from build123d import *

# Parameters (mm, degrees)
SKETCH_1_R          = 1.75
EXTRUDE_1_DEPTH     = 6
FILLET_1_R          = 3
SKETCH_2_R          = 0.5
CUT_EXTRUDE_1_DEPTH = 7


with BuildPart() as part:
    # Эскиз1 → Бобышка-Вытянуть1 (new body)
    with BuildSketch(Plane(origin=(0, 0, 0), x_dir=(1, 0, 0), z_dir=(0, 1, 0))):
        with BuildLine():
            Line((-3.991673782, 0), (4.008326218, 0))
            ThreePointArc((4.008326218, 0), (5.472792312, 3.535533906), (9.008326218, 5))
            Line((9.008326218, 5), (22.681786604, 5))
            ThreePointArc((22.681786604, 5), (25.510213728, 3.828427125), (26.681786604, 1))
            Line((26.681786604, 1), (29.008326218, 1))
            Line((29.008326218, 1), (53.280650212, 9.83440345))
            ThreePointArc((53.280650212, 9.83440345), (56.269012599, 16.242967271), (49.860448779, 19.231329658))
            Line((49.860448779, 19.231329658), (27.245056411, 11))
            Line((27.245056411, 11), (4.445056411, 11))
            ThreePointArc((4.445056411, 11), (-1.63962848, 6.931421506), (-3.991673782, 0))
        make_face()
        with Locations((51.570549496, 14.532866554)):
            Circle(SKETCH_1_R, mode=Mode.SUBTRACT)
        with Locations((29.781786604, 6)):
            Circle(SKETCH_1_R, mode=Mode.SUBTRACT)
    extrude(amount=EXTRUDE_1_DEPTH)

    # Скругление1
    fillet_1_edges = [part.edges().sort_by_distance(p)[0] for p in [
        (29.008326218, 3, -1),
    ]]
    fillet(fillet_1_edges, radius=FILLET_1_R)

    # Эскиз2 → Вырез-Вытянуть1 (cut, through all)
    with BuildSketch(Plane(origin=(0, 6, 0), x_dir=(1, 0, 0), z_dir=(0, 1, 0))):
        with Locations((1.008326218, 0)):
            Circle(SKETCH_2_R)
        with Locations((3.008326218, 0)):
            Circle(SKETCH_2_R)
        with Locations((-0.991673782, 0)):
            Circle(SKETCH_2_R)
        with Locations((-2.991673782, 0)):
            Circle(SKETCH_2_R)
    extrude(amount=-CUT_EXTRUDE_1_DEPTH, mode=Mode.SUBTRACT)


solid = part.part
Design review of the part built by this model. Coordinates are the model's own, in mm. A direction names the side the tool comes from. Coordinates: 2 decimals unless noted, no trailing zeros. Loops run counter-clockwise (first coordinate to the right, second up) from the corner with the lowest first, then second, coordinate; pieces in that order, holes last.
Item 1: Draft analysis for pull direction X (two halves, no side actions). For faces 4 (the flat face through (16, 3, -11)), 5 (the flat face through (38.711, 2.958, -15.173)), 6 (the cylindrical face through (-3, 3, -0.5)), state which applies: pulls with the +X half, pulls with the -X half, needs draft (parallel to the pull), parting line crosses it, or undercut.
Completed:
face 4: needs draft
face 5: pulls with the -X half
face 6: undercut
Item 2: Add section B-B (x = 13.5). Write out the cut boundary in (y, z).
Completed:
outline: (0, -11) - (6, -11) - (6, -5) - (0, -5) - close
Item 3: For faces 1 (the flat face through (28, 3, -1)), 2 (the cylindrical face through (25.48, 2.96, -3.86)), 3 (the cylindrical face through (53.2, 3, -13.9)), list the 3-axis set-ups (+Z, -Z, +X, -X, +Y, -Y) from which the entire face can be reached by the end or side of a thin tool; tool diameter is ignored.
Completed:
face 1: +Z, +X, +Y, -Y
face 2: +Z, +Y, -Y
face 3: +Y, -Y
Item 4: Add section D-D (x = 34.5). Write out the cut boundary in (y, z).
Completed:
outline: (0, -13.64) - (6, -13.64) - (6, -3) - (0, -3) - close
Item 5: Add section C-C (y = 2.2). Write out the cut boundary in (x, z).
Completed:
outline: (-3.99, 0) arc R11.39 ccw to (4.45, -11) - (27.25, -11) - (49.86, -19.23) arc R5 ccw to (53.28, -9.83) - (29.51, -1.18) arc R3 ccw to (28.48, -1) - (26.68, -1) arc R4 cw to (22.68, -5) - (9.01, -5) arc R5 cw to (4.01, 0) - (3.51, 0) arc R0.5 cw to (2.51, 0) - (1.51, 0) arc R0.5 cw to (0.51, 0) - (-0.49, 0) arc R0.5 cw to (-1.49, 0) - (-2.49, 0) arc R0.5 cw to (-3.49, 0) - close; hole circle Ø3.5 at (29.78, -6); hole circle Ø3.5 at (51.57, -14.53)
Item 6: Clearance check with flat-ended pins moving along their axes: pin 1 (3 mm diameter, centred on x = 15.5, y = 2.5, fed in from +Z); pin 2 (1.4 mm diameter, centred on x = 27.5, y = 2, fed in from +Z); pin 3 (1 mm diameter, centred on x = 42.5, z = -14.5, fed in from -Y); pin 4 (3 mm diameter, centred on y = 5, z = -12, fed in from -X). State where each tip first meets the part, or that it passes through.
Completed:
pin 1: stops at z = -5
pin 2: stops at z = -1
pin 3: stops at y = 0
pin 4: stops at x = 2.99
Item 7: Add section A-A (z = -7). Write out the cut boundary in (x, y), and give its area (3 significant figures).
Completed:
outline: (-1.59, 0) - (28.35, 0) - (28.35, 6) - (-1.59, 6) - close; (31.22, 0) - (45.49, 0) - (45.49, 6) - (31.22, 6) - close
area: 265 mm2
Item 8: Wall thickness on L1, parallel to Z at x = 53, y = 0.5; L2, parallel to Z at x = 2, y = 4.7; L3, parallel to Z at x = 45, y = 4.6: over which ranges is each line inside the solid? List them lowest first.
Completed:
L1: z = -19.32 to -15.54, -13.52 to -9.73
L2: z = -10.03 to 0
L3: z = -17.46 to -6.82
